The figure shows three views and two pictorial views of one solid part (mm, origin at its lowest corner). Answer the questions. A direction names the side the tool comes from. Give positions to 0.01 mm unless a question says otherwise; leave off trailing zeros. Order: outer loops, then holes, each group sorted by start corner. A loop starts at its lowest first (then second) coordinate and runs counter-clockwise, first axis right, second up. Notation, with made-up numbers: (-17, 70) - (19, 70) arc R36 cw to (19, 109) - close; hole circle Ø10 at (-34, 23.25). An arc over 180 degrees is marked (long way). Answer as a JSON object with one key per item and string values. Group by question number.
Q1. A cutting plane is placed at C-C, the plane z = 11. Give the vertices of the cut face in (x, y) (3 decimals), and give its area (3 significant figures).
Q2. A cutting plane is placed at D-D, the plane x = 1.5. Give the vertices of the cut face in (y, z), and give its area (3 significant figures).
Q3. The mould has two halves that part along Y. Classify the marked faces 4, 5 and 6: released by +Y, released by -Y, zero draft, split by the parting line, or undercut.
Q4. A cutting plane is placed at A-A, the plane y = 4. Give the vertices of the cut face in (x, z) (3 decimals), and give its area (4 significant figures).
Q5. Consider line 1 (Y direction, x = 4, z = 2) (3 decimals); line 2 (Y direction, x = 4, z = 6) (3 decimals); line 3 (X direction, y = 2.75, z = 0.5). Determine where each line is inside the solid, lowest interval first.
Q6. Given pin 1 (1.5 mm diameter, centred on y = 7, z = 7, fed in from -X); pin 2 (1 mm diameter, centred on y = 1.5, z = 3, fed in from +X); pin 3 (3 mm diameter, centred on x = 4, y = 5, fed in from -Z); pin 4 (1 mm diameter, centred on x = 3.5, y = 3.5, fed in from -Z), each flat-ended and moving along its own axis, determine where each tip first touches the part or whether it passes through.
Q7. For the marked faces 1, 2 and 3, determine the directions among +Z, -Z, +X, -X, +Y, -Y from which every point of the face is accessible in a straight line to the end or side of a thin tool.
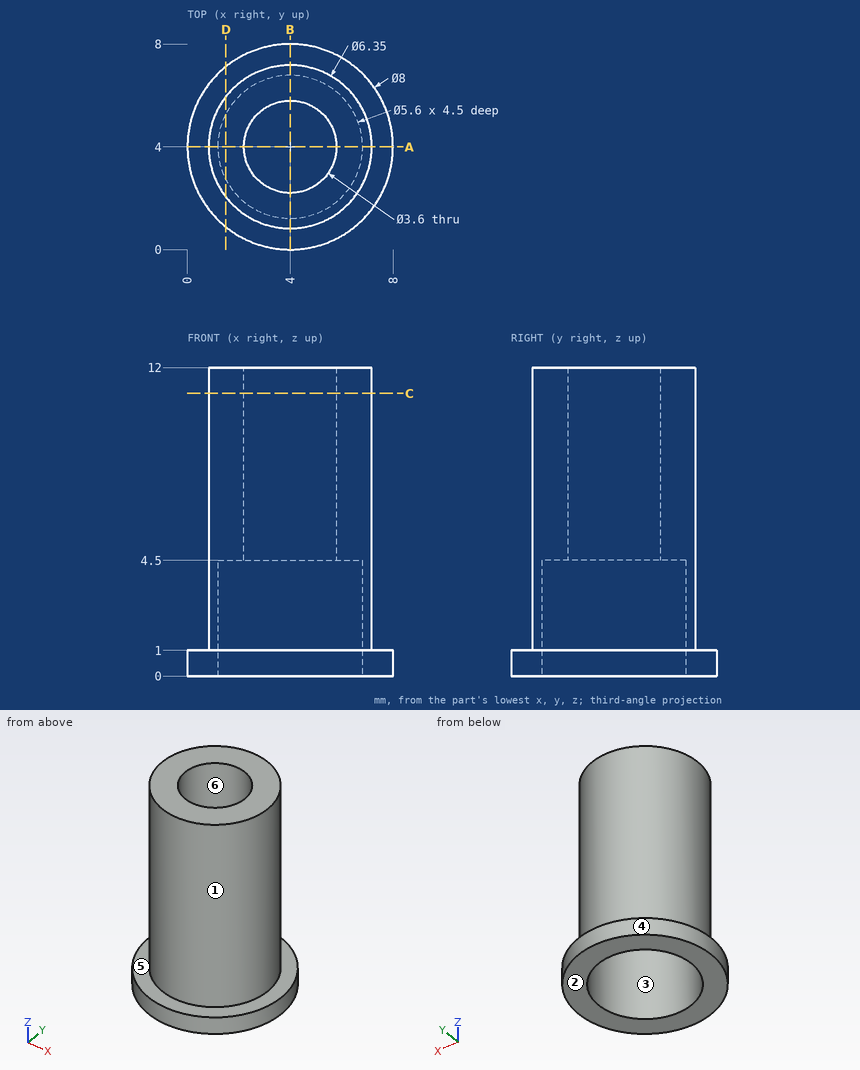
Reply:
{
 "1": {"outline": "circle Ø6.35 at (4, 4); hole circle Ø3.6 at (4, 4)", "area": "21.5 mm^2"},
 "2": {"outline": "(0.88, 0) - (2.74, 0) - (2.74, 4.5) - (5.26, 4.5) - (5.26, 0) - (7.12, 0) - (7.12, 1) - (5.96, 1) - (5.96, 12) - (2.04, 12) - (2.04, 1) - (0.88, 1) - close", "area": "38.0 mm^2"},
 "3": {"face 4": "split by the parting line", "face 5": "zero draft", "face 6": "undercut"},
 "4": {"outline": "(0, 0) - (1.2, 0) - (1.2, 4.5) - (2.2, 4.5) - (2.2, 12) - (0.825, 12) - (0.825, 1) - (0, 1) - close; (5.8, 4.5) - (6.8, 4.5) - (6.8, 0) - (8, 0) - (8, 1) - (7.175, 1) - (7.175, 12) - (5.8, 12) - close", "area": "25.65 mm^2"},
 "5": {"line 1": "y = 0.825 to 1.2, 6.8 to 7.175", "line 2": "y = 0.825 to 2.2, 5.8 to 7.175", "line 3": "x = 0.2 to 1.49, 6.51 to 7.8"},
 "6": {"pin 1": "stops at x = 1.76", "pin 2": "stops at x = 6.47", "pin 3": "stops at z = 4.5", "pin 4": "passes through"},
 "7": {"face 1": "+Z", "face 2": "-Z, +X, -X, +Y, -Y", "face 3": "-Z"}
}
